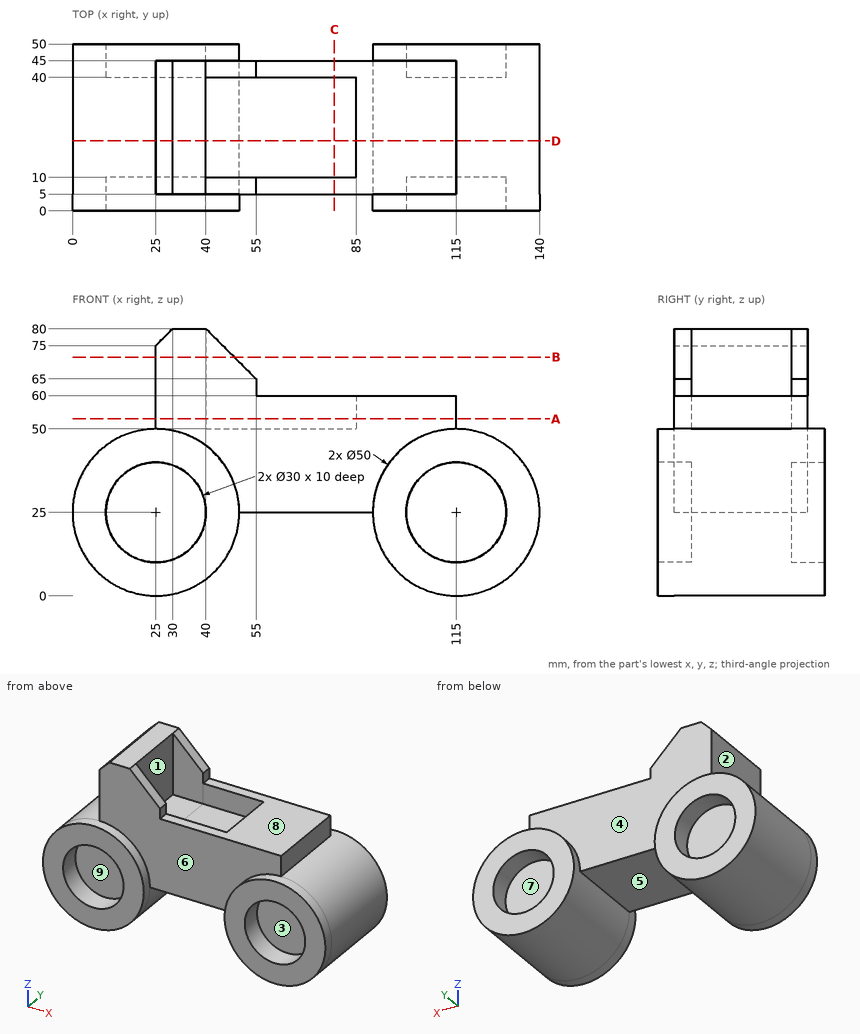
Part print with two shaded views. Sizes in mm from the minimum x, y, z corner. A direction names the side the tool comes from. Round coordinates to 2 decimals unless told otherwise and drop trailing zeros. Order: outer loops, then holes, each group sorted by start corner. A loop starts at its lowest first (then second) coordinate and runs counter-clockwise, first axis right, second up. Notation, with made-up numbers: (9.5, 35.25) -> (60.5, 35.25) arc R7 cw to (60.5, 42.25) -> close; hole circle Ø7 at (46.25, 66). An arc over 180 degrees is marked (long way). Use one line per item in the form item = value.
Item 1: Cut at C-C, the plane x = 78.5. Write the cut outline in (y, z), and give its area (3 significant figures).
Returned:
outline = (5, 25) -> (45, 25) -> (45, 60) -> (40, 60) -> (40, 50) -> (10, 50) -> (10, 60) -> (5, 60) -> close
area = 1,100 mm^2
Item 2: Cut at A-A, the plane z = 53. Write the cut outline in (x, y), and give its area (3 significant figures).
Returned:
outline = (25, 5) -> (115, 5) -> (115, 45) -> (25, 45) -> close; hole (40, 10) -> (85, 10) -> (85, 40) -> (40, 40) -> close
area = 2,250 mm^2
Item 3: Cut at B-B, the plane z = 71.5. Write the cut outline in (x, y), and give its area (3 significant figures).
Returned:
outline = (25, 5) -> (48.5, 5) -> (48.5, 10) -> (40, 10) -> (40, 40) -> (48.5, 40) -> (48.5, 45) -> (25, 45) -> close
area = 685 mm^2
Item 4: Pull direction Z, two halves, no side cores. Call the marked faces 6, 7, 8 and 9: released by +Z, released by -Z, zero draft, split by the parting line, or undercut.
Returned:
face_6 = zero draft
face_7 = undercut
face_8 = released by +Z
face_9 = undercut
Item 5: Tool access for the marked faces 1, 2, 3, 4 and 5: list every direction of +Z, -Z, +X, -X, +Y, -Y with a clear straight run to the whole face (end or side of a thin tool).
Returned:
face_1 = +Z
face_2 = +Z, -X, +Y, -Y
face_3 = -Y
face_4 = +Z, +Y
face_5 = -Z, +Y, -Y
Item 6: Drill centre lines: line 1 (X direction, y = 17, z = 59); line 2 (Y direction, x = 47, z = 58); line 3 (X direction, y = 7.5, z = 36.5). Where is each one in solid material? Low to high.
Returned:
line_1 = 25 to 40, 85 to 115
line_2 = 5 to 10, 40 to 45
line_3 = 2.8 to 15.37, 34.63 to 105.37, 124.63 to 137.2
Item 7: Flat gauge pins, fed straight in: pin 1 Ø9 at (x, z) = (109, 32) entering from -Y; pin 2 Ø12 at (y, z) = (30, 60.5) entering from -X; pin 3 Ø5.5 at (y, z) = (8, 61.5) entering from +X. Where does each tip first touch, or does it go through?
Returned:
pin_1 = 10
pin_2 = 25
pin_3 = 115
Item 8: Cut at D-D, the plane y = 21. Write the cut outline in (x, z), and give its area (3 significant figures).
Returned:
outline = (25, 50) arc R25 ccw (long way) to (50, 25) -> (90, 25) arc R25 ccw (long way) to (115, 50) -> (115, 60) -> (85, 60) -> (85, 50) -> (40, 50) -> (40, 80) -> (30, 80) -> (25, 75) -> close
area = 5,930 mm^2
